The model under review builds one solid part; all positions refer to its coordinate system, in mm. Face numbers are marked on the shaded views. A direction names the side the tool comes from. Coordinates: 2 decimals unless noted, no trailing zeros. Write each loop counter-clockwise with the first axis right and the second up, starting at its lowest first coordinate (ties: lowest second). Pieces come first, ordered by that corner, then holes.
1) For P1, Ø5, axis at y = 8.5, z = 7.5, coming from the -X side; P2, Ø0.7, axis at y = 24.5, z = 1.5, coming from the +X side, all flat-tipped, find the tip position at first contact; note any pin that passes through.
2) For line 1 (Y direction, x = 24, z = 6.5); line 2 (Z direction, x = 65.5, y = 5); line 3 (X direction, y = 24, z = -4.5), list the stretches that pass through material, from the lowest coordinate up.
3) Machinability: for the marked faces 1, 2 and 3, which of the approach directions +Z, -Z, +X, -X, +Y, -Y give a long, thin tool a straight path to every point of the face, cutting with its end or side? Answer none if there is none.
4) Add section C-C, the plane y = 12.75. State the section outline as (x, z) points, then the cut area to 3 significant figures.
5) Mouldability with a two-part tool opening along Z and no side actions: class the marked faces 4, 5 and 6 as released by +Z, released by -Z, zero draft, split by the parting line, or undercut.
6) Add section A-A, the plane x = 102.5. State the section outline as (y, z) points.
7) Add section B-B, the plane z = 6.5. State the section outline as (x, y) points, then the cut area to 3 significant figures.
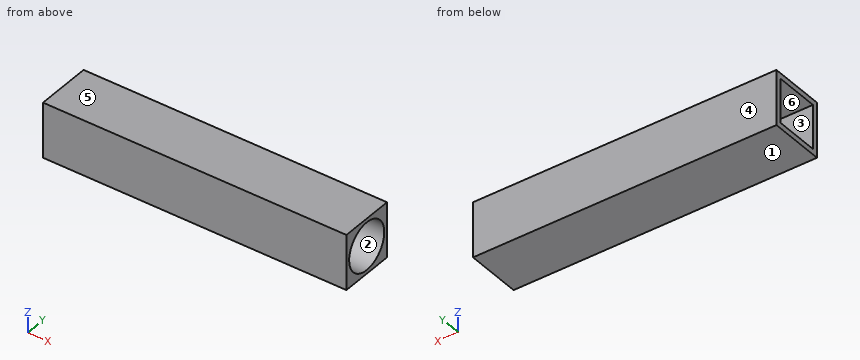
Autodesk Inventor part; units mm, degrees
ref_plane "YZ Plane" through (0, 0, 0) normal (1, 0, 0) x (0, 1, 0)
ref_plane "XZ Plane" through (0, 0, 0) normal (0, 1, 0) x (-1, 0, 0)
ref_plane "XY Plane" through (0, 0, 0) normal (0, 0, 1) x (1, 0, 0)
sketch "Sketch1" plane through (0, 0, 0) normal (1, 0, 0) x (0, 1, 0)
  line L0 (1.2978, 13.4356) -> (26.6978, 13.4356)
  line L1 (26.6978, 13.4356) -> (26.6978, -11.9644)
  line L2 (26.6978, -11.9644) -> (1.2978, -11.9644)
  line L3 (1.2978, -11.9644) -> (1.2978, 13.4356)
  line L4 (24.1578, -9.4244) -> (24.1578, 10.8956)
  line L5 (24.1578, 10.8956) -> (3.8378, 10.8956)
  line L6 (3.8378, 10.8956) -> (3.8378, -9.4244)
  line L7 (3.8378, -9.4244) -> (24.1578, -9.4244)
  point P0 (0, 0)
  dimension "d0" = 25.4
  dimension "d1" = 25.4
  dimension "d2" = 2.54
extrude "Extrusion1" add sketch "Sketch1" along normal blind 139.7
sketch "Sketch2" plane through (0, 3.8378, -9.4244) normal (0, 0, 1) x (1, 0, 0)
  line L0 (0, 0) -> (139.7, 0)
  line L1 (139.7, 0) -> (118.618, 0)
  line L2 (118.618, 0) -> (118.618, 20.32)
  line L3 (118.618, 20.32) -> (139.7, 20.32)
  line L4 (139.7, 20.32) -> (139.7, 0)
  point P0 (0, -3.8378)
  dimension "d5" = 21.082
  dimension "d6" = 20.32
extrude "Extrusion2" add sketch "Sketch2" along normal blind 20.32
sketch "Sketch3" plane through (139.7, 0, 0) normal (1, 0, 0) x (0, 0, -1)
  line L0 (11.9644, 1.2978) -> (-13.4356, 1.2978)
  line L1 (-0.7356, 1.2978) -> (-0.7356, 13.9978)
  line L2 (-13.4356, 26.6978) -> (11.9644, 26.6978)
  circle A0 centre (-0.7356, 13.9978) radius 10.9855
  point P0 (0, 0)
  dimension "d9" = 12.7
  dimension "d10" = 21.971
extrude "Extrusion3" cut sketch "Sketch3" against normal blind 21.082
thread "Thread1"
properties part number "2nd arm"
Geometry results:
1. P1: stops at x = 118.62
1. P2: stops at x = 118.62
2. line 1: y = 1.3 to 3.84, 24.16 to 26.7
2. line 2: z = -11.96 to -9.42, 10.9 to 13.44
2. line 3: x = 118.62 to 139.7
3. face 1: -Z, +X, -X, +Y, -Y
3. face 2: +X
3. face 3: -X
4. outline: (0, -11.96) - (139.7, -11.96) - (139.7, -10.18) - (118.62, -10.18) - (118.62, -9.42) - (0, -9.42) - close; (0, 10.9) - (118.62, 10.9) - (118.62, 11.65) - (139.7, 11.65) - (139.7, 13.44) - (0, 13.44) - close
4. area: 678 mm2
5. face 4: zero draft
5. face 5: released by +Z
5. face 6: undercut
6. outline: (1.3, -11.96) - (26.7, -11.96) - (26.7, 13.44) - (1.3, 13.44) - close; hole (3.84, -9.42) - (24.16, -9.42) - (24.16, 10.9) - (3.84, 10.9) - close
7. outline: (0, 1.3) - (139.7, 1.3) - (139.7, 4.65) - (118.62, 4.65) - (118.62, 3.84) - (0, 3.84) - close; (0, 24.16) - (118.62, 24.16) - (118.62, 23.35) - (139.7, 23.35) - (139.7, 26.7) - (0, 26.7) - close
7. area: 744 mm2
